For this review, take the finished solid that the model builds, in its own axes (mm). Face numbers are marked on the shaded views. A direction names the side the tool comes from. Coordinates: 2 decimals unless noted, no trailing zeros. Loops run counter-clockwise (first coordinate to the right, second up) from the corner with the lowest first, then second, coordinate; pieces in that order, holes last.
```python
from build123d import *

# Parameters (mm, degrees)
SKETCH1_W            = 45
SKETCH1_H            = 50
BOSS_EXTRUDE1_DEPTH  = 16
CUT_EXTRUDE1_DEPTH   = 58.116109812
SKETCH4_W            = 24
SKETCH4_H            = 50
CUT_EXTRUDE2_DEPTH   = 0.72
CUT_EXTRUDE3_DEPTH   = 58.116109812
SKETCH8_R            = 7.5
CUT_EXTRUDE4_DEPTH   = 0.72
M6_CLEARANCE_HOLE2_D = 7
CUT_EXTRUDE5_DEPTH   = 2.5
FILLET1_R            = 1
FILLET2_R            = 1
FILLET4_R            = 0.5
CUT_EXTRUDE7_DEPTH   = 11.5
SKETCH18_R           = 2.75
CUT_EXTRUDE8_DEPTH   = 14.5
SKETCH19_R           = 2.75
CUT_EXTRUDE9_DEPTH   = 10
SKETCH21_W           = 8.99
SKETCH21_H           = 50
BOSS_EXTRUDE2_DEPTH  = 0.6
CHAMFER1_SIZE        = 4
FILLET5_R            = 1
CUT_EXTRUDE11_DEPTH  = 4
CHAMFER2_SIZE        = 1


with BuildPart() as part:
    # Sketch1 → Boss-Extrude1 (new body)
    with BuildSketch(Plane(origin=(0, 0, 0), x_dir=(1, 0, 0), z_dir=(0, 1, 0))):
        Rectangle(SKETCH1_W, SKETCH1_H)
    extrude(amount=BOSS_EXTRUDE1_DEPTH)

    # Sketch3 → Cut-Extrude1 (cut, through all)
    with BuildSketch(Plane.XY.offset(25)):
        Polygon((-13.5, 16), (-17.5, 12), (22.5, 12), (22.5, 16), align=None)
    extrude(amount=-CUT_EXTRUDE1_DEPTH, mode=Mode.SUBTRACT)

    # Sketch4 → Cut-Extrude2 (cut)
    with BuildSketch(Plane(origin=(0, 12, 0), x_dir=(1, 0, 0), z_dir=(0, 1, 0))):
        with Locations((2.5, 0)):
            Rectangle(SKETCH4_W, SKETCH4_H)
    extrude(amount=-CUT_EXTRUDE2_DEPTH, mode=Mode.SUBTRACT)

    # Sketch5 → Cut-Extrude3 (cut, through all)
    with BuildSketch(Plane.XY.offset(25)):
        Polygon((-22.5, 16), (-13.5, 16), (-13.51, 15.99), (-22.5, 15.99), align=None)
    extrude(amount=-CUT_EXTRUDE3_DEPTH, mode=Mode.SUBTRACT)

    # Sketch8 → Cut-Extrude4 (cut)
    with BuildSketch(Plane(origin=(0, 11.28, 0), x_dir=(1, 0, 0), z_dir=(0, 1, 0))):
        with Locations(Location((2.5, 0, 0), (0, 0, 180))):
            Circle(SKETCH8_R)
    extrude(amount=-CUT_EXTRUDE4_DEPTH, mode=Mode.SUBTRACT)

    # M6 Clearance Hole2 (through all)
    with Locations(Plane(origin=(0, 10.56, 0), x_dir=(1, 0, 0), z_dir=(0, 1, 0))):
        with Locations((2.5, 0)):
            Hole(M6_CLEARANCE_HOLE2_D / 2)

    # Sketch12 → Cut-Extrude5 (cut)
    with BuildSketch(Plane(origin=(0, 11.28, 0), x_dir=(1, 0, 0), z_dir=(0, 1, 0))):
        with BuildLine():
            Line((7.5, 16.6), (-2.5, 16.6))
            ThreePointArc((-2.5, 16.6), (-3.207106781, 16.892893219), (-3.5, 17.6))
            Line((-3.5, 17.6), (-3.5, 25))
            Line((-3.5, 25), (8.5, 25))
            Line((8.5, 25), (8.5, 17.6))
            ThreePointArc((8.5, 17.6), (8.207106781, 16.892893219), (7.5, 16.6))
        make_face()
    cut_extrude5 = extrude(amount=-CUT_EXTRUDE5_DEPTH, mode=Mode.SUBTRACT)

    # Fillet1
    fillet1_edges = [part.edges().sort_by_distance(p)[0] for p in [
        (-3.5, 10.03, -25),
        (8.5, 10.03, -25),
    ]]
    fillet(fillet1_edges, radius=FILLET1_R)

    # Mirror2: Cut-Extrude5 across plane
    add(cut_extrude5.mirror(Plane.XY), mode=Mode.SUBTRACT)

    # Fillet2
    # the kernel refuses this fillet: 1 mm, written as the material it takes off along each edge
    with BuildSketch(Plane(origin=(7.5, 11.28, 17.6), x_dir=(1, 0, 0), z_dir=(0, 0, 1))) as fillet2_piece_1:
        with BuildLine():
            CenterArc((1 + FILLET2_R, -FILLET2_R), FILLET2_R, 90, 90)
            Line((1, -FILLET2_R), (1 - FILLET2_R * 0.02, -FILLET2_R))
            Line((1 - FILLET2_R * 0.02, -FILLET2_R), (1 - FILLET2_R * 0.02, FILLET2_R * 0.02))
            Line((1 - FILLET2_R * 0.02, FILLET2_R * 0.02), (1 + FILLET2_R, FILLET2_R * 0.02))
            Line((1 + FILLET2_R, FILLET2_R * 0.02), (1 + FILLET2_R, 0))
        make_face()
    revolve(axis=Axis((7.5, 11.28, 17.6), (0, 1, 0)), revolution_arc=90, mode=Mode.SUBTRACT)
    with BuildSketch(Plane(origin=(8.5, 11.28, 27.5), x_dir=(1, 0, 0), z_dir=(0, 0, -1)), Plane(origin=(-3.5, 11.28, 17.6), x_dir=(-1, 0, 0), z_dir=(0, 0, 1))) as fillet2_piece_2:
        with BuildLine():
            CenterArc((FILLET2_R, FILLET2_R), FILLET2_R, 180, 90)
            Line((0, FILLET2_R), (-FILLET2_R * 0.02, FILLET2_R))
            Line((-FILLET2_R * 0.02, FILLET2_R), (-FILLET2_R * 0.02, -FILLET2_R * 0.02))
            Line((-FILLET2_R * 0.02, -FILLET2_R * 0.02), (FILLET2_R, -FILLET2_R * 0.02))
            Line((FILLET2_R, -FILLET2_R * 0.02), (FILLET2_R, 0))
        make_face()
    extrude(amount=9.9, mode=Mode.SUBTRACT)
    with BuildSketch(Plane(origin=(-2.5, 11.28, 17.6), x_dir=(0, 0, -1), z_dir=(1, 0, 0))) as fillet2_piece_3:
        with BuildLine():
            CenterArc((1 + FILLET2_R, -FILLET2_R), FILLET2_R, 90, 90)
            Line((1, -FILLET2_R), (1 - FILLET2_R * 0.02, -FILLET2_R))
            Line((1 - FILLET2_R * 0.02, -FILLET2_R), (1 - FILLET2_R * 0.02, FILLET2_R * 0.02))
            Line((1 - FILLET2_R * 0.02, FILLET2_R * 0.02), (1 + FILLET2_R, FILLET2_R * 0.02))
            Line((1 + FILLET2_R, FILLET2_R * 0.02), (1 + FILLET2_R, 0))
        make_face()
    revolve(axis=Axis((-2.5, 11.28, 17.6), (0, 1, 0)), revolution_arc=90, mode=Mode.SUBTRACT)
    with BuildSketch(Plane(origin=(7.5, 11.28, 16.6), x_dir=(0, 0, -1), z_dir=(-1, 0, 0))) as fillet2_piece_4:
        with BuildLine():
            CenterArc((FILLET2_R, FILLET2_R), FILLET2_R, 180, 90)
            Line((0, FILLET2_R), (-FILLET2_R * 0.02, FILLET2_R))
            Line((-FILLET2_R * 0.02, FILLET2_R), (-FILLET2_R * 0.02, -FILLET2_R * 0.02))
            Line((-FILLET2_R * 0.02, -FILLET2_R * 0.02), (FILLET2_R, -FILLET2_R * 0.02))
            Line((FILLET2_R, -FILLET2_R * 0.02), (FILLET2_R, 0))
        make_face()
    extrude(amount=10, mode=Mode.SUBTRACT)
    with BuildSketch(Plane(origin=(-4.5, 11.28, -25), x_dir=(0, 0, 1), z_dir=(-1, 0, 0)), Plane(origin=(14.5, 11.28, -25), x_dir=(0, 0, 1), z_dir=(-1, 0, 0))) as fillet2_piece_5:
        with BuildLine():
            CenterArc((FILLET2_R, -FILLET2_R), FILLET2_R, 90, 90)
            Line((0, -FILLET2_R), (-FILLET2_R * 0.02, -FILLET2_R))
            Line((-FILLET2_R * 0.02, -FILLET2_R), (-FILLET2_R * 0.02, FILLET2_R * 0.02))
            Line((-FILLET2_R * 0.02, FILLET2_R * 0.02), (FILLET2_R, FILLET2_R * 0.02))
            Line((FILLET2_R, FILLET2_R * 0.02), (FILLET2_R, 0))
        make_face()
    extrude(amount=5, mode=Mode.SUBTRACT)
    with BuildSketch(Plane(origin=(2.5, 11.28, 0), x_dir=(-1, 0, 0), z_dir=(0, 0, -1))) as fillet2_piece_6:
        with BuildLine():
            CenterArc((8.46, -1), FILLET2_R, 90, 73.739795292)
            Line((7.5, -0.72), (7.4808, -0.7144))
            ThreePointArc((7.4808, -0.7144), (7.48, -0.36), (7.48, 0))
            Line((7.48, 0), (7.5, 0.02))
            Line((7.5, 0.02), (8.46, 0.02))
            Line((8.46, 0.02), (8.46, 0))
        make_face()
    revolve(axis=Axis((2.5, 11.28, 0), (0, 1, 0)), mode=Mode.SUBTRACT)
    with BuildSketch(Plane(origin=(7.5, 11.28, -17.6), x_dir=(1, 0, 0), z_dir=(0, 0, -1))) as fillet2_piece_7:
        with BuildLine():
            CenterArc((1 + FILLET2_R, FILLET2_R), FILLET2_R, 180, 90)
            Line((1, FILLET2_R), (1 - FILLET2_R * 0.02, FILLET2_R))
            Line((1 - FILLET2_R * 0.02, FILLET2_R), (1 - FILLET2_R * 0.02, -FILLET2_R * 0.02))
            Line((1 - FILLET2_R * 0.02, -FILLET2_R * 0.02), (1 + FILLET2_R, -FILLET2_R * 0.02))
            Line((1 + FILLET2_R, -FILLET2_R * 0.02), (1 + FILLET2_R, 0))
        make_face()
    revolve(axis=Axis((7.5, 11.28, -17.6), (0, -1, 0)), revolution_arc=90, mode=Mode.SUBTRACT)
    with BuildSketch(Plane(origin=(8.5, 11.28, -24), x_dir=(1, 0, 0), z_dir=(0, 0, 1)), Plane(origin=(-3.5, 11.28, -17.6), x_dir=(-1, 0, 0), z_dir=(0, 0, -1))) as fillet2_piece_8:
        with BuildLine():
            CenterArc((FILLET2_R, -FILLET2_R), FILLET2_R, 90, 90)
            Line((0, -FILLET2_R), (-FILLET2_R * 0.02, -FILLET2_R))
            Line((-FILLET2_R * 0.02, -FILLET2_R), (-FILLET2_R * 0.02, FILLET2_R * 0.02))
            Line((-FILLET2_R * 0.02, FILLET2_R * 0.02), (FILLET2_R, FILLET2_R * 0.02))
            Line((FILLET2_R, FILLET2_R * 0.02), (FILLET2_R, 0))
        make_face()
    extrude(amount=6.4, mode=Mode.SUBTRACT)
    with BuildSketch(Plane(origin=(-2.5, 11.28, -17.6), x_dir=(0, 0, 1), z_dir=(1, 0, 0))) as fillet2_piece_9:
        with BuildLine():
            CenterArc((1 + FILLET2_R, FILLET2_R), FILLET2_R, 180, 90)
            Line((1, FILLET2_R), (1 - FILLET2_R * 0.02, FILLET2_R))
            Line((1 - FILLET2_R * 0.02, FILLET2_R), (1 - FILLET2_R * 0.02, -FILLET2_R * 0.02))
            Line((1 - FILLET2_R * 0.02, -FILLET2_R * 0.02), (1 + FILLET2_R, -FILLET2_R * 0.02))
            Line((1 + FILLET2_R, -FILLET2_R * 0.02), (1 + FILLET2_R, 0))
        make_face()
    revolve(axis=Axis((-2.5, 11.28, -17.6), (0, -1, 0)), revolution_arc=90, mode=Mode.SUBTRACT)
    with BuildSketch(Plane(origin=(7.5, 11.28, -16.6), x_dir=(0, 0, 1), z_dir=(-1, 0, 0))) as fillet2_piece_10:
        with BuildLine():
            CenterArc((FILLET2_R, -FILLET2_R), FILLET2_R, 90, 90)
            Line((0, -FILLET2_R), (-FILLET2_R * 0.02, -FILLET2_R))
            Line((-FILLET2_R * 0.02, -FILLET2_R), (-FILLET2_R * 0.02, FILLET2_R * 0.02))
            Line((-FILLET2_R * 0.02, FILLET2_R * 0.02), (FILLET2_R, FILLET2_R * 0.02))
            Line((FILLET2_R, FILLET2_R * 0.02), (FILLET2_R, 0))
        make_face()
    extrude(amount=10, mode=Mode.SUBTRACT)
    with BuildSketch(Plane(origin=(-4.5, 11.28, -24), x_dir=(0, 0, -1), z_dir=(-1, 0, 0))) as fillet2_piece_11:
        with BuildLine():
            CenterArc((1 - FILLET2_R, FILLET2_R), FILLET2_R, 270, 90)
            Line((1, FILLET2_R), (1 + FILLET2_R * 0.02, FILLET2_R))
            Line((1 + FILLET2_R * 0.02, FILLET2_R), (1 + FILLET2_R * 0.02, 0))
            Line((1 + FILLET2_R * 0.02, 0), (1, -FILLET2_R * 0.02))
            Line((1, -FILLET2_R * 0.02), (1 - FILLET2_R, -FILLET2_R * 0.02))
            Line((1 - FILLET2_R, -FILLET2_R * 0.02), (1 - FILLET2_R, 0))
        make_face()
    revolve(axis=Axis((-4.5, 11.28, -24), (0, -1, 0)), revolution_arc=90, mode=Mode.SUBTRACT)
    with BuildSketch(Plane(origin=(9.5, 11.28, -24), x_dir=(0, 0, -1), z_dir=(1, 0, 0))) as fillet2_piece_12:
        with BuildLine():
            CenterArc((1 - FILLET2_R, -FILLET2_R), FILLET2_R, 0, 90)
            Line((1, -FILLET2_R), (1 + FILLET2_R * 0.02, -FILLET2_R))
            Line((1 + FILLET2_R * 0.02, -FILLET2_R), (1 + FILLET2_R * 0.02, 0))
            Line((1 + FILLET2_R * 0.02, 0), (1, FILLET2_R * 0.02))
            Line((1, FILLET2_R * 0.02), (1 - FILLET2_R, FILLET2_R * 0.02))
            Line((1 - FILLET2_R, FILLET2_R * 0.02), (1 - FILLET2_R, 0))
        make_face()
    revolve(axis=Axis((9.5, 11.28, -24), (0, 1, 0)), revolution_arc=90, mode=Mode.SUBTRACT)

    # Fillet4
    fillet4_edges = [part.edges().sort_by_distance(p)[0] for p in [
        (-17.5, 12, 0),
    ]]
    fillet(fillet4_edges, radius=FILLET4_R)

    # Sketch14 → Cut-Extrude7 (cut)
    with BuildSketch(Plane(origin=(0, 12, 0), x_dir=(1, 0, 0), z_dir=(0, 1, 0))):
        Polygon((19.5, -8), (17.5, -8), (17.5, -3.45), (16.1, -3.45), (16.1, 3.45), (17.5, 3.45), (17.5, 8), (19.5, 8), align=None)
    extrude(amount=-CUT_EXTRUDE7_DEPTH, mode=Mode.SUBTRACT)

    # Sketch18 → Cut-Extrude8 (cut)
    with BuildSketch(Plane(origin=(22.5, 0, 0), x_dir=(0, 0, -1), z_dir=(1, 0, 0))):
        with Locations((0, 6)):
            Circle(SKETCH18_R)
    extrude(amount=-CUT_EXTRUDE8_DEPTH, mode=Mode.SUBTRACT)

    # Sketch19 → Cut-Extrude9 (cut)
    with BuildSketch(Plane(origin=(22.5, 0, 0), x_dir=(0, 0, -1), z_dir=(1, 0, 0))):
        with Locations((-16, 6)):
            Circle(SKETCH19_R)
        with Locations((16, 6)):
            Circle(SKETCH19_R)
    extrude(amount=-CUT_EXTRUDE9_DEPTH, mode=Mode.SUBTRACT)

    # Sketch21 → Boss-Extrude2 (add)
    with BuildSketch(Plane(origin=(0, 15.99, 0), x_dir=(1, 0, 0), z_dir=(0, 1, 0))):
        with Locations((-18.005, 0)):
            Rectangle(SKETCH21_W, SKETCH21_H)
    extrude(amount=BOSS_EXTRUDE2_DEPTH)

    # Chamfer1
    chamfer1_edges = [part.edges().sort_by_distance(p)[0] for p in [
        (-22.5, 8.295, 25),
        (-22.5, 8.295, -25),
    ]]
    chamfer(chamfer1_edges, length=CHAMFER1_SIZE)

    # Fillet5
    fillet5_edges = [part.edges().sort_by_distance(p)[0] for p in [
        (-22.5, 16.59, 0),
    ]]
    fillet(fillet5_edges, radius=FILLET5_R)

    # Sketch23 → Cut-Extrude11 (cut)
    with BuildSketch(Plane(origin=(0, 10.56, 0), x_dir=(1, 0, 0), z_dir=(0, 1, 0))):
        Polygon((2.5, 6.618818118), (-3.232064633, 3.309409059), (-3.232064633, -3.309409059), (2.5, -6.618818118), (8.232064633, -3.309409059), (8.232064633, 3.309409059), align=None)
    extrude(amount=-CUT_EXTRUDE11_DEPTH, mode=Mode.SUBTRACT)

    # Chamfer2
    chamfer2_edges = [part.edges().sort_by_distance(p)[0] for p in [
        (18.5, 12, 8),
        (18.5, 12, -8),
    ]]
    chamfer(chamfer2_edges, length=CHAMFER2_SIZE)


solid = part.part
```
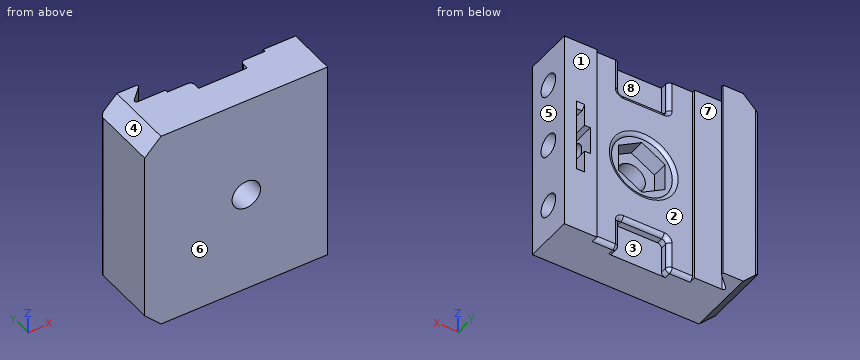
Q1. Machinability: for the marked faces 1, 2, 3 and 4, which of the approach directions +Z, -Z, +X, -X, +Y, -Y give a long, thin tool a straight path to every point of the face, cutting with its end or side? Answer none if there is none.
Q2. For pin 1 Ø1.2 at (y, z) = (9.5, 22.5) entering from -X; pin 2 Ø6 at (y, z) = (13.5, -2.5) entering from +X; pin 3 Ø12 at (x, z) = (3.5, -3) entering from +Y; pin 4 Ø9 at (x, z) = (20, -6) entering from +Y, all flat-tipped, find the tip position at first contact; note any pin that passes through.
Q3. Consider section D-D (y = 14). State the section outline as (x, z) points.
Q4. Consider section B-B (z = 0). Count the separate pieces of the cut face and the enclosed holes in it, then the cut area to 3 significant figures.
Q5. The part is to be moulded in two halves that separate along Y. For the marked faces 5, 6, 7 and 8, say which applies: +Y half, -Y half, draft (parallel to the pull), parting line (faces both ways), or undercut.
Q6. Consider section C-C (x = -7.5). State the section outline as (y, z) points.
Q7. Wall thickness on probe 1 along X at (y, z) = (8.5, 1.5); probe 2 along X at (y, z) = (11.75, 4); probe 3 along X at (y, z) = (6.5, 4): over which ranges is each line inside the solid? List them lowest first.
Model answer:
1. face 1: +Z, -Z, +X, +Y
1. face 2: +Z, -Z, +Y
1. face 3: -Z, +Y
1. face 4: +Z, -X, +Y, -Y
2. pin 1: stops at x = -21.6
2. pin 2: stops at x = 22.5
2. pin 3: stops at y = 11.28
2. pin 4: stops at y = 12
3. outline: (-22.5, -21) - (-18.5, -25) - (-15.5, -25) - (-15.5, 25) - (-18.5, 25) - (-22.5, 21) - close
4. separate pieces: 4
4. enclosed holes: 0
4. area: 354 mm2
5. face 5: draft
5. face 6: -Y half
5. face 7: undercut
5. face 8: +Y half
6. outline: (0, -25) - (10.28, -25) arc R1 ccw to (11.28, -24) - (11.28, 25) - (0, 25) - close
7. probe 1: x = -22.5 to -3.23, 8.23 to 16.1, 19.5 to 22.5
7. probe 2: x = -22.5 to -9.5, 14.5 to 17.5, 19.5 to 22.5
7. probe 3: x = -22.5 to 17.5, 19.5 to 22.5
